from build123d import *

# Parameters (mm, degrees)
SKETCH_2_W          = 43.1785014
SKETCH_2_H          = 22.86
EXTRUDE_1_DEPTH     = 1.6
SKETCH_3_R          = 1.283879863
SKETCH_3_R_2        = 1.281760523
SKETCH_3_R_3        = 1.2500102
CUT_EXTRUDE_1_DEPTH = 1.6
EXTRUDE_2_DEPTH     = 1
EXTRUDE_3_DEPTH     = 0.5
SKETCH_6_R          = 2.445789306
EXTRUDE_4_DEPTH     = 4
EXTRUDE_5_DEPTH     = 0.1
SKETCH_9_W          = 2.815880296
SKETCH_9_H          = 1.422027446
SKETCH_9_H_2        = 1.462665737
SKETCH_9_W_2        = 2.865727124
SKETCH_9_H_3        = 1.505721031
SKETCH_9_H_4        = 1.440958836
EXTRUDE_6_DEPTH     = 0.8
SKETCH_10_W         = 2.7701748
SKETCH_10_H         = 1.3212064
EXTRUDE_7_DEPTH     = 0.5
FILLET_1_R          = 4


with BuildPart() as part:
    # 草图2 → 凸台-拉伸1 (new body)
    with BuildSketch(Plane.XY):
        with Locations((20.3207493, 10.16)):
            Rectangle(SKETCH_2_W, SKETCH_2_H)
    extrude(amount=EXTRUDE_1_DEPTH)

    # 草图3 → 切除-拉伸1 (cut)
    with BuildSketch(Plane.XY.offset(1.6)):
        with Locations((2.5414986, 17.7785014)):
            Circle(SKETCH_3_R)
        with Locations((2.54, 2.54)):
            Circle(SKETCH_3_R_2)
        with Locations((38.227, 2.54)):
            Circle(SKETCH_3_R_2)
        with Locations((38.1, 17.78)):
            Circle(SKETCH_3_R_3)
    extrude(amount=-CUT_EXTRUDE_1_DEPTH, mode=Mode.SUBTRACT)

    # 草图4 → 凸台-拉伸2 (add)
    with BuildSketch(Plane.XY.offset(1.6)):
        with BuildLine():
            Line((32.004, 14.945995), (33.3149956, 14.945995))
            Line((33.3149956, 14.945995), (33.3149956, 9.946005))
            Line((33.3149956, 9.946005), (28.9150044, 9.946005))
            Line((28.9150044, 9.946005), (28.9150044, 14.945995))
            Line((28.9150044, 14.945995), (30.226, 14.945995))
            ThreePointArc((30.226, 14.945995), (31.115, 14.056677443), (32.004, 14.945995))
        make_face()
    extrude(amount=EXTRUDE_2_DEPTH)

    # 草图5 → 凸台-拉伸3 (add)
    with BuildSketch(Plane.XY.offset(1.6)):
        Polygon((11.3538, 13.28166), (9.95934, 11.8872), (9.95934, 6.53034), (16.711168, 6.529832), (16.711168, 11.8860316), (15.3150316, 13.282168), align=None)
        Polygon((18.4658, 13.28166), (17.07134, 11.8872), (17.07134, 6.53034), (23.823168, 6.529832), (23.823168, 11.8860316), (22.4270316, 13.282168), align=None)
    extrude(amount=EXTRUDE_3_DEPTH)

    # 草图6 → 凸台-拉伸4 (add)
    with BuildSketch(Plane.XY.offset(2.1)):
        with Locations((13.335, 9.752040279)):
            Circle(SKETCH_6_R)
        with Locations((20.4464158, 9.752040279)):
            Circle(SKETCH_6_R)
    extrude(amount=EXTRUDE_4_DEPTH)

    # 草图7 → 凸台-拉伸5 (add)
    with BuildSketch(Plane.XY.offset(1.6)):
        with BuildLine():
            Line((1.397, 11.417275077), (3.683, 11.417275077))
            ThreePointArc((3.683, 11.417275077), (4.940275077, 10.16), (3.683, 8.902724923))
            Line((3.683, 8.902724923), (1.397, 8.902724923))
            ThreePointArc((1.397, 8.902724923), (0.139724923, 10.16), (1.397, 11.417275077))
        make_face()
        with BuildLine():
            Line((1.384057208, 14.463336619), (3.670057208, 14.463336619))
            ThreePointArc((3.670057208, 14.463336619), (4.927332285, 13.206061542), (3.670057208, 11.948786466))
            Line((3.670057208, 11.948786466), (1.384057208, 11.948786466))
            ThreePointArc((1.384057208, 11.948786466), (0.126782131, 13.206061542), (1.384057208, 14.463336619))
        make_face()
        with BuildLine():
            Line((1.384057208, 8.530334061), (3.670057208, 8.530334061))
            ThreePointArc((3.670057208, 8.530334061), (4.927332285, 7.273058984), (3.670057208, 6.015783908))
            Line((3.670057208, 6.015783908), (1.384057208, 6.015783908))
            ThreePointArc((1.384057208, 6.015783908), (0.126782131, 7.273058984), (1.384057208, 8.530334061))
        make_face()
        with BuildLine():
            Line((35.801623871, 9.688824593), (38.087623871, 9.688824593))
            ThreePointArc((38.087623871, 9.688824593), (39.344898948, 8.431549516), (38.087623871, 7.17427444))
            Line((38.087623871, 7.17427444), (35.801623871, 7.17427444))
            ThreePointArc((35.801623871, 7.17427444), (34.544348794, 8.431549516), (35.801623871, 9.688824593))
        make_face()
        with BuildLine():
            Line((26.408339557, 19.359447221), (26.408339557, 16.596292633))
            ThreePointArc((26.408339557, 16.596292633), (25.197327361, 15.385280436), (23.986315165, 16.596292633))
            Line((23.986315165, 16.596292633), (23.986315165, 19.359447221))
            ThreePointArc((23.986315165, 19.359447221), (25.197327361, 20.570459417), (26.408339557, 19.359447221))
        make_face()
    extrude(amount=EXTRUDE_5_DEPTH)

    # 草图9 → 凸台-拉伸6 (add)
    with BuildSketch(Plane.XY.offset(1.6)):
        with Locations((37.32890041, 14.350017877)):
            Rectangle(SKETCH_9_W, SKETCH_9_H)
        with Locations((37.32890041, 12.569367647)):
            Rectangle(SKETCH_9_W, SKETCH_9_H_2)
        with Locations((25.644961239, 10.555802193)):
            Rectangle(SKETCH_9_W_2, SKETCH_9_H_3)
        with Locations((25.644961239, 8.726270188)):
            Rectangle(SKETCH_9_W_2, SKETCH_9_H_4)
    extrude(amount=EXTRUDE_6_DEPTH)

    # 草图10 → 凸台-拉伸7 (add)
    with BuildSketch(Plane.XY.offset(1.6)):
        with Locations((30.988, 16.891)):
            Rectangle(SKETCH_10_W, SKETCH_10_H)
    extrude(amount=EXTRUDE_7_DEPTH)

    # 圆角1
    fillet_1_edges = [part.edges().sort_by_distance(p)[0] for p in [
        (-1.2685014, 21.59, 0.8),
        (41.91, 21.59, 0.8),
        (41.91, -1.27, 0.8),
        (-1.2685014, -1.27, 0.8),
    ]]
    fillet(fillet_1_edges, radius=FILLET_1_R)


solid = part.part
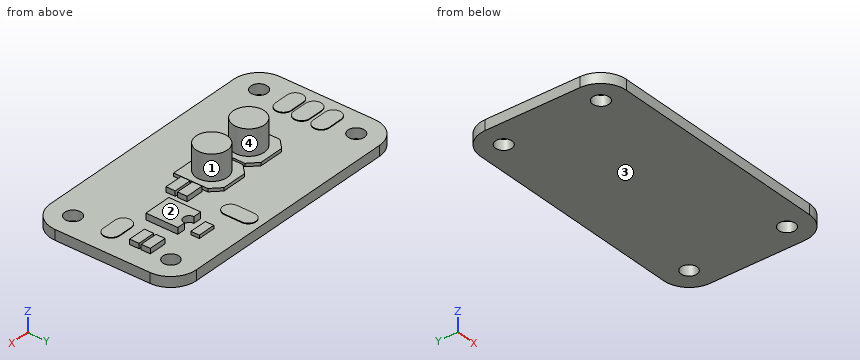
Can you work these out from the model? Positions are in its coordinate system, mm. Face numbers are marked on the shaded views. A direction names the side the tool comes from. Give positions to 0.01 mm unless a question says otherwise; leave off trailing zeros. Loops run counter-clockwise (first coordinate to the right, second up) from the corner with the lowest first, then second, coordinate; pieces in that order, holes last. Notation, with made-up numbers: (40.25, -27) - (95.25, -27) arc R37 ccw to (95.25, 11) - close; hole circle Ø5 at (15.25, 82). An arc over 180 degrees is marked (long way). Return JSON: item names as keys, results as strings.
1. I want a section at C-C on y = 5. Please give me the cut outline in (x, z).
Output values:
{"outline": "(-1.27, 0) - (41.91, 0) - (41.91, 1.6) - (-1.27, 1.6) - close"}
2. I'm going to push flat-ended pins straight in: pin 1 Ø3.5 at (x, y) = (31.5, 13) entering from +Z; pin 2 Ø1.5 at (y, z) = (10, 5) entering from +X; pin 3 Ø2 at (x, y) = (3, 13) entering from +Z. Where does each tip first touch, or does it pass through?
Output values:
{"pin 1": "stops at z = 2.6", "pin 2": "stops at x = 22.89", "pin 3": "stops at z = 1.7"}
3. For the marked faces 3 and 4, which set-ups out of +Z, -Z, +X, -X, +Y, -Y let a thin tool reach every point of the face, with its end or its side?
Output values:
{"face 3": "-Z, +X, -X, +Y, -Y", "face 4": "+Z"}
4. I want a section at B-B on x = 20. Please give me the cut outline in (y, z).
Output values:
{"outline": "(-1.27, 0) - (21.59, 0) - (21.59, 1.6) - (13.28, 1.6) - (13.28, 2.1) - (12.16, 2.1) - (12.16, 6.1) - (7.35, 6.1) - (7.35, 2.1) - (6.53, 2.1) - (6.53, 1.6) - (-1.27, 1.6) - close"}
5. I want a section at A-A on x = 2. Please give me the cut outline in (y, z), and give its area (3 significant figures).
Output values:
{"outline": "(-1.2, 0) - (1.38, 0) - (1.38, 1.6) - (-1.2, 1.6) - close; (3.7, 0) - (16.61, 0) - (16.61, 1.6) - (14.46, 1.6) - (14.46, 1.7) - (11.95, 1.7) - (11.95, 1.6) - (11.42, 1.6) - (11.42, 1.7) - (8.9, 1.7) - (8.9, 1.6) - (8.53, 1.6) - (8.53, 1.7) - (6.02, 1.7) - (6.02, 1.6) - (3.7, 1.6) - close; (18.94, 0) - (21.52, 0) - (21.52, 1.6) - (18.94, 1.6) - close", "area": "29.7 mm²"}
6. We'd pull the mould along X, two halves only. Please class the marked faces 1 and 2: +X half, -X half, draft (parallel to the pull), parting line (faces both ways), or undercut.
Output values:
{"face 1": "undercut", "face 2": "draft"}
7. If I drill on line 1 (Y direction, x = 38.1, z = 1.1); line 2 (X direction, y = 9, z = 2.25); line 3 (Z direction, x = 7.5, y = 19.25), over which ranges is the centre line in solid material (lowest first)?
Output values:
{"line 1": "y = -1.27 to 1.26, 3.82 to 16.53, 19.03 to 21.59", "line 2": "x = 11.01 to 15.66, 18.12 to 22.77, 24.21 to 27.08", "line 3": "z = 0 to 1.6"}
8. I want a section at D-D on z = 5. Please give me the cut outline in (x, y) (3 decimals).
Output values:
{"outline": "circle Ø4.892 at (13.335, 9.752); circle Ø4.892 at (20.446, 9.752)"}
